Source: CAD feature listing. Evaluate the final solid. Frame: model axes, mm. A direction names the side the tool comes from. Give positions to 0.01 mm unless a question says otherwise; leave off trailing zeros. Order: outer loops, then holes, each group sorted by start corner. A loop starts at its lowest first (then second) coordinate and runs counter-clockwise, first axis right, second up.
1) Draft query along Z for faces 1 (the face through (0, 1.5, 0)), 2 (the face through (0, 16, -10)), 3 (the face through (0, 0, 0)), 4 (the face through (-0.21, 0.54, -10.98)). Return one class per face: released by +Z, released by -Z, zero draft, split by the parting line, or undercut.
2) Section B-B, the plane x = 9.25. Return loops of the section in (y, z).
3) First-contact query: P1, Ø9.5, axis at x = 5.5, z = 0, coming from the +Y side; P2, Ø10, axis at y = 8, z = -2, coming from the -X side. Flat tips, straight axial feed; report the tip coordinate or a pass-through.
4) Section C-C, the plane z = -2.25. Return loops of the section in (x, y), plus the area to 3 significant figures.
5) Section A-A, the plane y = 4.75. Return loops of the section in (x, z), plus the area to 3 significant figures.
6) Material intervals for line 1 (Z direction, x = -3, y = 15.75); line 2 (Y direction, x = -4.75, z = 9.5), sorted ascending.
7) Access query for faces 5 (the face through (0, 16, 10)), 6 (the face through (0, 30, 11)). Directions: +Z, -Z, +X, -X, +Y, -Y. A direction counts if a zero-diameter tool reaches every point of the face in a straight line with its end or side. Return the directions, or none.
Autodesk Inventor part; units mm, degrees
ref_plane "YZ Plane" through (0, 0, 0) normal (1, 0, 0) x (0, 1, 0)
ref_plane "XZ Plane" through (0, 0, 0) normal (0, 1, 0) x (-1, 0, 0)
ref_plane "XY Plane" through (0, 0, 0) normal (0, 0, 1) x (1, 0, 0)
sketch "Sketch1" plane through (0, 0, 0) normal (0, 1, 0) x (-1, 0, 0)
  line L0 (-15, 10) -> (15, 10)
  line L1 (15, 10) -> (15, -10)
  line L2 (15, -10) -> (-15, -10)
  line L3 (-15, -10) -> (-15, 10)
  line L4 (-15, 10) -> (15, -10) construction
  line L5 (15, 10) -> (-15, -10) construction
  point P0 (0, 0)
  dimension "d0" = 20
  dimension "d1" = 30
extrude "Plate1" add sketch "Sketch1" along normal blind 1.5
sketch "Sketch2" plane through (-15, 0, -11.5) normal (0, 0, 1) x (1, 0, 0)
  line L0 (30, 0) -> (0, 0)
  line L1 (0, 0) -> (0, 30)
  line L2 (0, 30) -> (30, 30)
  line L3 (30, 30) -> (30, 0)
edge flange "Flange1" height 30 angle 90 thickness 1.5 bend radius 0.31 thickness toward (0, 0, 1) relief tear relief width 1.5 relief depth 0.75 corner gap 0.31 corner form 0 edges at (0, 1.5, -10) (0, 1.5, 10) wall of the first edge with corners at (15, 0, -11.5) (-15, 0, -11.5) (-15, 30, -11.5) (15, 30, -11.5)
bend "Bend1"
corner "Corner1"
equation "\"d2\" = Thickness"
equation "\"d3\" = BendReliefWidth"
equation "\"d4\" = BendReliefDepth"
equation "\"d5\" = MinimumRemnant"
equation "\"d6\" = TransitionRadius"
equation "\"d9\" = BendRadius"
equation "\"d10\" = CornerReliefSize"
equation "\"d11\" = GapSize"
equation "\"d12\" = JacobiRadiusSize"
equation "\"BendReliefWidth\" = Thickness"
equation "\"BendReliefDepth\" = 0.5 * Thickness"
equation "\"CornerReliefSize\" = 4 * Thickness"
equation "\"MinimumRemnant\" = 2 * Thickness"
equation "\"TransitionRadius\" = BendRadius"
equation "\"JacobiRadiusSize\" = BendRadius"
equation "\"GapSize\" = Thickness"
properties part number "axis_19_top_frame" material "Aluminum 6061-AHC"
From the geometry:
1. face 1: undercut
1. face 2: undercut
1. face 3: zero draft
1. face 4: released by -Z
2. outline: (0, -9.69) arc R1.81 ccw to (1.81, -11.5) - (30, -11.5) - (30, -10) - (1.81, -10) arc R0.31 cw to (1.5, -9.69) - (1.5, 9.69) arc R0.31 cw to (1.81, 10) - (30, 10) - (30, 11.5) - (1.81, 11.5) arc R1.81 ccw to (0, 9.69) - close
3. P1: stops at y = 1.5
3. P2: passes through
4. outline: (-15, 0) - (15, 0) - (15, 1.5) - (-15, 1.5) - close
4. area: 45.0 mm2
5. outline: (-15, -11.5) - (15, -11.5) - (15, -10) - (-15, -10) - close; (-15, 10) - (15, 10) - (15, 11.5) - (-15, 11.5) - close
5. area: 90.0 mm2
6. line 1: z = -11.5 to -10, 10 to 11.5
6. line 2: y = 0 to 1.5
7. face 5: +X, -X, +Y
7. face 6: +Z, -Z, +X, -X, +Y
